Read the model definition and answer for the solid it produces. Units are mm, in the model's axes. Face numbers are marked on the shaded views. A direction names the side the tool comes from. Give positions to 0.01 mm unless a question says otherwise; leave off trailing zeros. Write each loop counter-clockwise with the first axis right and the second up, starting at its lowest first coordinate (ties: lowest second). Pieces come first, ordered by that corner, then holes. Notation, with made-up numbers: (0, -4) - (58, -4) arc R18 ccw to (58, 14) - close; hole circle Ø3 at (55, -13.75). An arc over 180 degrees is marked (long way). Use CSV: the item, a comma, the result in double quotes. Start each with the question number.
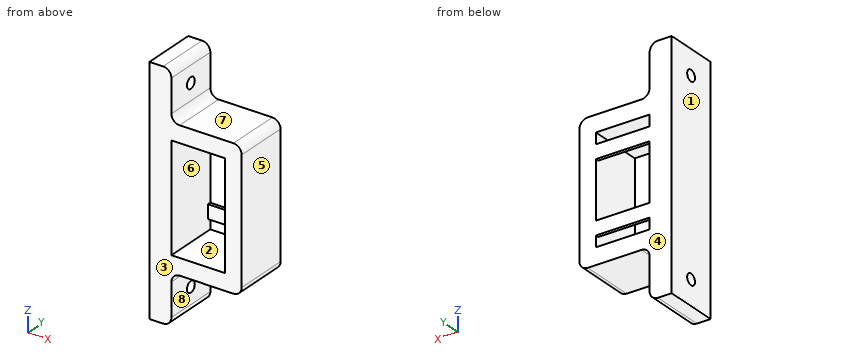
from build123d import *

# Parameters (mm, degrees)
F1_DEPTH = 20
F2_W     = 19.6
F2_H     = 38.7
F3_DEPTH = 25
F4_R     = 2
F5_DEPTH = 25
F6_W     = 1.2
F6_H     = 5
F7_DEPTH = 19.6


with BuildPart() as f1:
    # F0 (on Front) → F1 (new body)
    with BuildSketch(Plane.XZ):
        with BuildLine():
            Line((-5.8, -25.35), (13.8, -25.35))
            ThreePointArc((13.8, -25.35), (15.92132, -24.47132), (16.8, -22.35))
            Line((16.8, -22.35), (16.8, 22.35))
            ThreePointArc((16.8, 22.35), (15.92132, 24.47132), (13.8, 25.35))
            Line((13.8, 25.35), (-5.8, 25.35))
            ThreePointArc((-5.8, 25.35), (-7.92132, 26.22868), (-8.8, 28.35))
            Line((-8.8, 28.35), (-8.8, 40.35))
            ThreePointArc((-8.8, 40.35), (-9.67868, 42.47132), (-11.8, 43.35))
            Line((-11.8, 43.35), (-16.8, 43.35))
            Line((-16.8, 43.35), (-16.8, 25.35))
            Line((-16.8, 25.35), (-16.8, -25.35))
            Line((-16.8, -25.35), (-16.8, -43.35))
            Line((-16.8, -43.35), (-11.8, -43.35))
            ThreePointArc((-11.8, -43.35), (-9.67868, -42.47132), (-8.8, -40.35))
            Line((-8.8, -40.35), (-8.8, -28.35))
            ThreePointArc((-8.8, -28.35), (-7.92132, -26.22868), (-5.8, -25.35))
        make_face()
    extrude(amount=F1_DEPTH)

    # F2 (on face) → F3 (cut)
    with BuildSketch(Plane.XZ.offset(20)):
        with Locations((1, 0)):
            Rectangle(F2_W, F2_H)
    extrude(amount=-F3_DEPTH, mode=Mode.SUBTRACT)

    # F4 (on face) → F5 (cut)
    with BuildSketch(Plane.YZ.offset(-8.8)):
        with Locations((-10, 34.35)):
            Circle(F4_R)
        with Locations((-10, -34.35)):
            Circle(F4_R)
    extrude(amount=-F5_DEPTH, mode=Mode.SUBTRACT)

    # F6 (on face) → F7 (join, through all)
    with BuildSketch(Plane.YZ.offset(-8.8)):
        with Locations((-0.6, 12.85)):
            Rectangle(F6_W, F6_H)
        with Locations((-0.6, -12.85)):
            Rectangle(F6_W, F6_H)
    extrude(amount=F7_DEPTH)


solid = f1.part
(1) Consider probe 1 along Z at (x, y) = (-13.75, -10); probe 2 along Z at (x, y) = (-11.5, -10); probe 3 along Z at (x, y) = (-6, -6.75). Determine where each line is inside the solid, lowest interval first.
(2) The part is cut by section C-C on x = 3.5. Write down the section's boundary in (y, z).
(3) The part is cut by section A-A on y = -10. Write down the section's boundary in (x, z), plus the area to 3 significant figures.
(4) Which of the six approach directions +Z, -Z, +X, -X, +Y, -Y give full straight-line access (tool end or side, diameter ignored) to the marked faces 4, 5, 6, 7 and 8?
(5) Given P1, Ø1, axis at x = 5.5, y = -0.5, coming from the -Z side; P2, Ø4, axis at x = -5, y = -5.5, coming from the -Z side; P3, Ø5.5, axis at x = 3.5, z = -12.5, coming from the -Y side, each flat-ended and moving along its own axis, determine where each tip first touches the part or whether it passes through.
(6) For a pull along X with two mould halves and no side action, classify the marked faces 1, 2 and 3 as pulls with the +X half, pulls with the -X half, needs draft (parallel to the pull), parting line crosses it, or undercut.
(7) The part is cut by section D-D on y = -14.75. Write down the section's boundary in (x, z).
(8) The part is cut by section B-B on z = 18. Write down the section's boundary in (x, y), plus the area to 3 significant figures.
Reported:
1,probe 1,"-43.35 to -36.35, -32.35 to 32.35, 36.35 to 43.35"
1,probe 2,"-43.33 to -36.35, -32.35 to 32.35, 36.35 to 43.33"
1,probe 3,"-25.36 to -19.35, 19.35 to 25.36"
2,outline,"(-20, -25.35) - (0, -25.35) - (0, -19.35) - (-20, -19.35) - close; (-20, 19.35) - (0, 19.35) - (0, 25.35) - (-20, 25.35) - close; (-1.2, -15.35) - (0, -15.35) - (0, -10.35) - (-1.2, -10.35) - close; (-1.2, 10.35) - (0, 10.35) - (0, 15.35) - (-1.2, 15.35) - close"
3,outline,"(-16.8, -43.35) - (-11.8, -43.35) arc R3 ccw to (-8.8, -40.35) - (-8.8, -36.35) - (-16.8, -36.35) - close; (-16.8, -32.35) - (-8.8, -32.35) - (-8.8, -28.35) arc R3 cw to (-5.8, -25.35) - (13.8, -25.35) arc R3 ccw to (16.8, -22.35) - (16.8, 22.35) arc R3 ccw to (13.8, 25.35) - (-5.8, 25.35) arc R3 cw to (-8.8, 28.35) - (-8.8, 32.35) - (-16.8, 32.35) - close; (-16.8, 36.35) - (-8.8, 36.35) - (-8.8, 40.35) arc R3 ccw to (-11.8, 43.35) - (-16.8, 43.35) - close; hole (-8.8, -19.35) - (10.8, -19.35) - (10.8, 19.35) - (-8.8, 19.35) - close"
3,area,"1,170 mm²"
4,face 4,"+Z, -Z, +X, -X, +Y"
4,face 5,"+Z, -Z, +X, +Y, -Y"
4,face 6,"-Y"
4,face 7,"+Z, +X, +Y, -Y"
4,face 8,"-Z, +X, +Y, -Y"
5,P1,"z = -25.35"
5,P2,"z = -25.6"
5,P3,"y = -1.2"
6,face 1,"pulls with the -X half"
6,face 2,"undercut"
6,face 3,"needs draft"
7,outline,"(-16.8, -43.35) - (-11.8, -43.35) arc R3 ccw to (-8.8, -40.35) - (-8.8, -28.35) arc R3 cw to (-5.8, -25.35) - (13.8, -25.35) arc R3 ccw to (16.8, -22.35) - (16.8, 22.35) arc R3 ccw to (13.8, 25.35) - (-5.8, 25.35) arc R3 cw to (-8.8, 28.35) - (-8.8, 40.35) arc R3 ccw to (-11.8, 43.35) - (-16.8, 43.35) - close; hole (-8.8, -19.35) - (10.8, -19.35) - (10.8, 19.35) - (-8.8, 19.35) - close"
8,outline,"(-16.8, -20) - (-8.8, -20) - (-8.8, 0) - (-16.8, 0) - close; (10.8, -20) - (16.8, -20) - (16.8, 0) - (10.8, 0) - close"
8,area,"280 mm²"
